```python
from build123d import *

# Parameters (mm, degrees)
SALIENTE_EXTRUIR1_DEPTH = 4
CORTAR_EXTRUIR1_REACH   = 131.701
CROQUIS4_W              = 4
CROQUIS4_H              = 30


with BuildPart() as part:
    # Croquis3 → Saliente-Extruir1 (new body)
    with BuildSketch(Plane(origin=(0, 0, 0), x_dir=(1, 0, 0), z_dir=(0, 1, 0))):
        Polygon((100, 82.5), (-100, 82.5), (-100, 62.5), (-62, 62.5), (-62, 2.5), (-100, 2.5), (-100, -82.5), (100, -82.5), (100, 2.5), (62, 2.5), (62, 62.5), (100, 62.5), align=None)
    extrude(amount=SALIENTE_EXTRUIR1_DEPTH)

    # Croquis4 → Cortar-Extruir1 (cut, up to next)
    with BuildSketch(Plane(origin=(0, 4, 0), x_dir=(1, 0, 0), z_dir=(0, 1, 0)), mode=Mode.PRIVATE) as cortar_extruir1_sk1:
        with Locations((98, -67.5)):
            Rectangle(CROQUIS4_W, CROQUIS4_H)
    cortar_extruir1_tool1 = extrude(cortar_extruir1_sk1.sketch, amount=-CORTAR_EXTRUIR1_REACH, mode=Mode.PRIVATE) & part.part
    # Croquis4 → Cortar-Extruir1 (cut, up to next)
    with BuildSketch(Plane(origin=(0, 4, 0), x_dir=(1, 0, 0), z_dir=(0, 1, 0)), mode=Mode.PRIVATE) as cortar_extruir1_sk2:
        with Locations((-98, -67.5)):
            Rectangle(CROQUIS4_W, CROQUIS4_H)
    cortar_extruir1_tool2 = extrude(cortar_extruir1_sk2.sketch, amount=-CORTAR_EXTRUIR1_REACH, mode=Mode.PRIVATE) & part.part
    add(cortar_extruir1_tool1.solids().sort_by_distance((98, 4, 67.5))[0], mode=Mode.SUBTRACT)
    add(cortar_extruir1_tool2.solids().sort_by_distance((-98, 4, 67.5))[0], mode=Mode.SUBTRACT)


solid = part.part
```
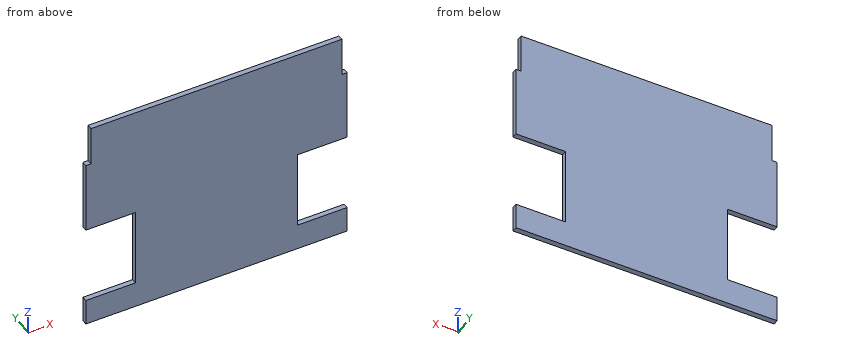
The listing builds one solid part. Answer for the finished solid, in the listing's coordinates (mm). Round coordinates to 2 decimals unless told otherwise and drop trailing zeros. Write each loop counter-clockwise with the first axis right and the second up, starting at its lowest first coordinate (ties: lowest second). Pieces come first, ordered by that corner, then holes. Notation, with made-up numbers: (10.5, 28.25) -> (25.5, 28.25) arc R9 cw to (25.5, 39.25) -> close; hole circle Ø9 at (-19, 88.25). An arc over 180 degrees is marked (long way). Answer as a JSON object with one key per item and string values. Group by question number.
Q1. Straight lines are drawn through the part: line 1 along Z through (x, y) = (91, 0.7); line 2 along X through (y, z) = (3.1, -61.5); line 3 along X through (y, z) = (3.7, 76.5). For each, find the intervals that lie inside material, in ascending order.
Q2. Each of these flat-tipped pins is pushed along its axis until it touches: pin 1 Ø1.5 at (y, z) = (0.5, -36.5) entering from -X; pin 2 Ø1.2 at (y, z) = (1, 62) entering from -X; pin 3 Ø1.2 at (y, z) = (2, -32.5) entering from +X. Where does it stop, or does it pass through?
Q3. Section A-A (y = 3) is taken. Write down the section's boundary in (x, z), plus the area to 3 significant figures.
Q4. Section B-B (z = -30.5) is taken. Write down the section's boundary in (x, y).
Check values:
{
 "1": {"line 1": "-82.5 to -62.5, -2.5 to 82.5", "line 2": "-62 to 62", "line 3": "-96 to 96"},
 "2": {"pin 1": "x = -62", "pin 2": "x = -96", "pin 3": "x = 62"},
 "3": {"outline": "(-100, -82.5) -> (100, -82.5) -> (100, -62.5) -> (62, -62.5) -> (62, -2.5) -> (100, -2.5) -> (100, 52.5) -> (96, 52.5) -> (96, 82.5) -> (-96, 82.5) -> (-96, 52.5) -> (-100, 52.5) -> (-100, -2.5) -> (-62, -2.5) -> (-62, -62.5) -> (-100, -62.5) -> close", "area": "28,200 mm^2"},
 "4": {"outline": "(-62, 0) -> (62, 0) -> (62, 4) -> (-62, 4) -> close"}
}
